Design review of the part built by this model. Coordinates are the model's own, in mm. Coordinates: 2 decimals unless noted, no trailing zeros. Loops run counter-clockwise (first coordinate to the right, second up) from the corner with the lowest first, then second, coordinate; pieces in that order, holes last. Notation, with made-up numbers: M 81,3.25 L 130,3.25 A10 cw 130,16.25 Z; hole C 50.25,30.25 d3. An arc over 180 degrees is marked long. Answer as a JSON object with one key per item and string values. Group by question number.
1. Consider section A-A (x = 0). State the section outline as (y, z) points.
2. Consider section B-B (z = 0). State the section outline as (x, y) points.
3. Insertion check: pin 1 (1 mm diameter, centred on x = -3, y = 2.5, fed in from +Z); pin 2 (2 mm diameter, centred on y = 2.5, z = 6, fed in from -X); pin 3 (1 mm diameter, centred on y = 2.5, z = 2.5, fed in from +X); pin 4 (8 mm diameter, centred on x = 0, z = 0, fed in from -Y). Each pin has a flat end and moves straight along its axis. Give the tip position at first contact, or say it passes through.
4. Draft analysis for pull direction X (two halves, no side actions). For faces 1 (the flat face through (2, 0, 5)), 2 (the cylindrical face through (1.08, 1.97, 4.88)), 3 (the cylindrical face through (7.493, 1.972, -0.33)), state which applies: +X half, -X half, draft (parallel to the pull), parting line (faces both ways), or undercut.
5. To check wall thickness, follow probe 1 along Z at (x, y) = (0, 0.1); probe 2 along X at (y, z) = (0.9, 2.25); probe 3 along X at (y, z) = (3.3, -3.75). State the ranges of each line that lie inside material, in increasing order.
6. Consider section D-D (x = 6.25). State the section outline as (y, z) points, then the cut area to 3 significant figures.
7. Consider section C-C (y = 0.85). State the section outline as (x, z) points.
Autodesk Inventor part; units mm, degrees
ref_plane "Work Plane1" through (0, 2, 0) normal (0, 1, 0) x (1, 0, 0)
ref_plane "YZ Plane" through (0, 0, 0) normal (1, 0, 0) x (0, 1, 0)
ref_plane "XZ Plane" through (0, 0, 0) normal (0, 1, 0) x (-1, 0, 0)
sketch "Sketch1" plane through (0, 0, 0) normal (0, 1, 0) x (-1, 0, 0)
  circle A0 centre (0, 0) radius 5
  circle A1 centre (0, 0) radius 7.5
  dimension "d0" = 10
  dimension "d1" = 15
extrude "Extrusion1" add sketch "Sketch1" along normal blind 4
sketch "Sketch2" plane through (0, 4, 0) normal (0, 1, 0) x (1, 0, 0)
  circle A0 centre (0, 0) radius 7.5
  circle A1 centre (0, 0) radius 5
  circle A2 centre (0, 0) radius 5.75
  circle A3 centre (0, 0) radius 6.75
  dimension "d4" = 11.5
  dimension "d5" = 13.5
extrude "Extrusion2" cut sketch "Sketch2" against normal blind 0.2 contours A3
ref_plane "Work Plane1" through (0, 2, 0) normal (0, 1, 0) x (1, 0, 0)
mirror "Mirror1" about plane through (0, 2, 0) normal (0, 1, 0) of "Extrusion2"
properties part number "bearing10X15X4"
Findings below:
{
 "1": {"outline": "M 0,-7.5 L 4,-7.5 L 4,-6.75 L 3.8,-6.75 L 3.8,-5.75 L 4,-5.75 L 4,-5 L 0,-5 L 0,-5.75 L 0.2,-5.75 L 0.2,-6.75 L 0,-6.75 Z; M 0,5 L 4,5 L 4,5.75 L 3.8,5.75 L 3.8,6.75 L 4,6.75 L 4,7.5 L 0,7.5 L 0,6.75 L 0.2,6.75 L 0.2,5.75 L 0,5.75 Z"},
 "2": {"outline": "M -7.5,0 L -6.75,0 L -6.75,0.2 L -5.75,0.2 L -5.75,0 L -5,0 L -5,4 L -5.75,4 L -5.75,3.8 L -6.75,3.8 L -6.75,4 L -7.5,4 Z; M 5,0 L 5.75,0 L 5.75,0.2 L 6.75,0.2 L 6.75,0 L 7.5,0 L 7.5,4 L 6.75,4 L 6.75,3.8 L 5.75,3.8 L 5.75,4 L 5,4 Z"},
 "3": {"pin 1": "stops at z = 7.07", "pin 2": "stops at x = -5.59", "pin 3": "stops at x = 7.23", "pin 4": "passes through"},
 "4": {"face 1": "draft", "face 2": "undercut", "face 3": "parting line"},
 "5": {"probe 1": "z = -7.5 to -6.75, -5.75 to -5, 5 to 5.75, 6.75 to 7.5", "probe 2": "x = -7.15 to -4.47, 4.47 to 7.15", "probe 3": "x = -6.5 to -3.31, 3.31 to 6.5"},
 "6": {"outline": "M 0,-4.15 L 4,-4.15 L 4,-2.55 L 3.8,-2.55 L 3.8,2.55 L 4,2.55 L 4,4.15 L 0,4.15 L 0,2.55 L 0.2,2.55 L 0.2,-2.55 L 0,-2.55 Z", "area": "31.1 mm^2"},
 "7": {"outline": "C 0,0 d15; hole C 0,0 d10"}
}
